```python
from build123d import *

# Parameters (mm, degrees)
BOSS_EXTRUDE1_DEPTH     = 15
M3_CLEARANCE_HOLE1_D    = 3.4
SKETCH4_R               = 1.5
CUT_EXTRUDE1_DEPTH      = 1
CUT_EXTRUDE1_DEPTH_BACK = 31


with BuildPart() as part:
    # Sketch1 → Boss-Extrude1 (new body, symmetric)
    with BuildSketch(Plane(origin=(0, 0, 0), x_dir=(0, 0, -1), z_dir=(1, 0, 0))):
        Polygon((-8, 8), (0, 8), (1, 8), (4, 5), (4, 3), (1, 0), (0, 0), (-6, 0), (-6, -8), (-8, -8), align=None)
    extrude(amount=BOSS_EXTRUDE1_DEPTH, both=True)

    # M3 Clearance Hole1 (through all)
    with Locations(Plane(origin=(0, 0, 6), x_dir=(-1, 0, 0), z_dir=(0, 0, -1))):
        with Locations((-10, -4), (10, -4)):
            Hole(M3_CLEARANCE_HOLE1_D / 2)

    # Sketch4 → Cut-Extrude1 (cut, two sides)
    with BuildSketch(Plane(origin=(15, 0, 0), x_dir=(0, 0, -1), z_dir=(1, 0, 0))) as cut_extrude1_sk:
        with Locations((0, 4)):
            Circle(SKETCH4_R)
    extrude(amount=CUT_EXTRUDE1_DEPTH, mode=Mode.SUBTRACT)
    extrude(cut_extrude1_sk.sketch, amount=-CUT_EXTRUDE1_DEPTH_BACK, mode=Mode.SUBTRACT)


solid = part.part
```
CAD build for the part. Positions are in the model's coordinates, mm. A direction names the side the tool comes from. Round coordinates to 2 decimals unless told otherwise and drop trailing zeros. Order: outer loops, then holes, each group sorted by start corner. A loop starts at its lowest first (then second) coordinate and runs counter-clockwise, first axis right, second up. Notation, with made-up numbers: (42.5, 7) - (75.5, 7) arc R14 cw to (75.5, 22) - close; hole circle Ø3 at (-0.5, 29.25). An arc over 180 degrees is marked (long way). Use CSV: the item, a comma, the result in double quotes. Start each with the question number.
1) Two-plate mould, pull along Z, no slides. Class faces 1 (the cylindrical face through (0.21, 5.265, -0.806)), 2 (the flat face through (0, 4, -4)), 3 (the flat face through (0, 0, 3)): pulls with the +Z half, pulls with the -Z half, needs draft (parallel to the pull), parting line crosses it, or undercut.
2) Tool access for faces 4 (the flat face through (0, -4, 6)), 5 (the cylindrical face through (-9.2, -5.5, 7)): list every direction of +Z, -Z, +X, -X, +Y, -Y with a clear straight run to the whole face (end or side of a thin tool).
3) Saw through at C-C (y = 4). List the corners of the cut face in (x, z), and give its area (3 significant figures).
4) Pin check, flat tips, straight feed: pin 1 Ø4.5 at (x, y) = (-10, -4) entering from -Z; pin 2 Ø5 at (x, z) = (-9.5, 0) entering from -Y; pin 3 Ø1.5 at (x, y) = (-2, 1.5) entering from -Z. Stop position of each tip, or through.
5) Saw through at A-A (y = -4). List the corners of the cut face in (x, z).
6) Wall check: L1, parallel to Y at x = 3, z = 0; L2, parallel to X at y = -5.5, z = 6.5; L3, parallel to Y at x = 10, z = 7.3. Give the ranges that are in metal, low to high. Write a range as [from, to].
7) Saw through at B-B (x = 10). List the corners of the cut face in (y, z), and give its area (3 significant figures).
8) Saw through at D-D (z = 0). List the corners of the cut face in (x, y), and give its area (3 significant figures).
Values follow:
1,face 1,"undercut"
1,face 2,"pulls with the -Z half"
1,face 3,"needs draft"
2,face 4,"-Z, +X, -X, -Y"
2,face 5,"+Z, -Z"
3,outline,"(-15, -4) - (15, -4) - (15, -1.5) - (-15, -1.5) - close; (-15, 1.5) - (15, 1.5) - (15, 8) - (-15, 8) - close"
3,area,"270 mm2"
4,pin 1,"stops at z = 6"
4,pin 2,"stops at y = 0"
4,pin 3,"stops at z = -3.25"
5,outline,"(-15, 6) - (-11.7, 6) - (-11.7, 8) - (-15, 8) - close; (-8.3, 6) - (8.3, 6) - (8.3, 8) - (-8.3, 8) - close; (11.7, 6) - (15, 6) - (15, 8) - (11.7, 8) - close"
6,L1,"y = [0, 2.5], [5.5, 8]"
6,L2,"x = [-15, -10.8], [-9.2, 9.2], [10.8, 15]"
6,L3,"y = [-8, -5.7], [-2.3, 8]"
7,outline,"(-8, 6) - (-5.7, 6) - (-5.7, 8) - (-8, 8) - close; (-2.3, 6) - (0, 6) - (0, -1) - (3, -4) - (5, -4) - (8, -1) - (8, 8) - (-2.3, 8) - close; hole circle Ø3 at (4, 0)"
7,area,"89.1 mm2"
8,outline,"(-15, 0) - (15, 0) - (15, 2.5) - (-15, 2.5) - close; (-15, 5.5) - (15, 5.5) - (15, 8) - (-15, 8) - close"
8,area,"150 mm2"
